```python
from build123d import *

# Parameters (mm, degrees)
SKETCH_1_R          = 14
EXTRUDE_1_DEPTH     = 19
SKETCH_2_W          = 13.202760332
SKETCH_2_H          = 6.2
EXTRUDE_2_DEPTH     = 15
SKETCH_3_R          = 1.75
EXTRUDE_3_DEPTH     = 1
SKETCH_4_R          = 4
EXTRUDE_4_DEPTH     = 1.8
SKETCH_5_R          = 2.5
EXTRUDE_5_DEPTH     = 8.2
CUT_EXTRUDE_START   = -6
CUT_EXTRUDE_1_DEPTH = 6


with BuildPart() as part:
    # 草图1 → 凸台-拉伸1 (new body)
    with BuildSketch(Plane(origin=(0, 0, 0), x_dir=(1, 0, 0), z_dir=(0, 1, 0))):
        with Locations(Location((0, 0, 0), (0, 0, 270))):
            Circle(SKETCH_1_R)
    extrude(amount=EXTRUDE_1_DEPTH)

    # 草图2 → 凸台-拉伸2 (add)
    with BuildSketch(Plane(origin=(0, 19, 0), x_dir=(1, 0, 0), z_dir=(0, 1, 0))):
        with Locations((0, -14)):
            Rectangle(SKETCH_2_W, SKETCH_2_H)
    extrude(amount=-EXTRUDE_2_DEPTH)

    # 草图3 → 凸台-拉伸3 (add)
    with BuildSketch(Plane(origin=(0, 19, 0), x_dir=(1, 0, 0), z_dir=(0, 1, 0))):
        with BuildLine():
            Line((17.5, -4), (-17.5, -4))
            ThreePointArc((-17.5, -4), (-21.5, 0), (-17.5, 4))
            Line((-17.5, 4), (17.5, 4))
            ThreePointArc((17.5, 4), (21.5, 0), (17.5, -4))
        make_face()
        with Locations(Location((-17.5, 0, 0), (0, 0, 270))):
            Circle(SKETCH_3_R, mode=Mode.SUBTRACT)
        with Locations(Location((17.5, 0, 0), (0, 0, 270))):
            Circle(SKETCH_3_R, mode=Mode.SUBTRACT)
    extrude(amount=-EXTRUDE_3_DEPTH)

    # 草图4 → 凸台-拉伸4 (add)
    with BuildSketch(Plane(origin=(0, 19, 0), x_dir=(1, 0, 0), z_dir=(0, 1, 0))):
        with Locations(Location((0, 6, 0), (0, 0, 270))):
            Circle(SKETCH_4_R)
    extrude(amount=EXTRUDE_4_DEPTH)

    # 草图5 → 凸台-拉伸5 (add)
    with BuildSketch(Plane(origin=(0, 20.8, 0), x_dir=(1, 0, 0), z_dir=(0, 1, 0))):
        with Locations(Location((0, 6, 0), (0, 0, 270))):
            Circle(SKETCH_5_R)
    extrude(amount=EXTRUDE_5_DEPTH)

    # 草图6 → 切除-拉伸1 (cut)
    with BuildSketch(Plane(origin=(0, 29, 0), x_dir=(1, 0, 0), z_dir=(0, 1, 0)).offset(CUT_EXTRUDE_START)):
        with BuildLine():
            Line((2, 4.5), (-2, 4.5))
            ThreePointArc((-2, 4.5), (0, 3.5), (2, 4.5))
        make_face()
        with BuildLine():
            Line((-2, 7.5), (2, 7.5))
            ThreePointArc((2, 7.5), (0, 8.5), (-2, 7.5))
        make_face()
    extrude(amount=CUT_EXTRUDE_1_DEPTH, mode=Mode.SUBTRACT)


solid = part.part
```
The model under review builds one solid part; all positions refer to its coordinate system, in mm. A direction names the side the tool comes from. Round coordinates to 2 decimals unless told otherwise and drop trailing zeros. Write each loop counter-clockwise with the first axis right and the second up, starting at its lowest first coordinate (ties: lowest second). Pieces come first, ordered by that corner, then holes.
(1) Machinability: for faces 4 (the cylindrical face through (-3.905, 19.887, -6.867)), 5 (the flat face through (0, 26, -7.5)), 6 (the flat face through (-15.5, 18.5, -4)), which of the approach directions +Z, -Z, +X, -X, +Y, -Y give a long, thin tool a straight path to every point of the face, cutting with its end or side? Answer none if there is none.
(2) We need section C-C on z = -6. Give the boundary of the cut face in (x, y).
(3) Mouldability with a two-part tool opening along Z and no side actions: class faces 1 (the cylindrical face through (2.11, 23.93, -4.66)), 2 (the cylindrical face through (19.235, 18.507, -0.228)), 3 (the flat face through (-15.4, 18.5, 4)) as +Z half, -Z half, draft (parallel to the pull), parting line (faces both ways), or undercut.
(4) We need section A-A on z = 0. Give the boundary of the cut face in (x, y).
(5) We need section B-B on x = 0. Give the boundary of the cut face in (y, z).
(6) We need section D-D on z = 6.5. Give the boundary of the cut face in (x, y), and give its area (3 significant figures).
(7) Wall thickness on L1, parallel to X at y = 18.5, z = 0; L2, parallel to Y at x = -12, z = 3; L3, parallel to X at y = 4.5, z = -10: over which ranges is each line inside the solid? List them lowest first.
(8) Insertion check: pin 1 (2 mm diameter, centred on y = 11.5, z = 2, fed in from -X); pin 2 (0.5 mm diameter, centred on x = 0, z = -8, fed in from +Y); pin 3 (0.8 mm diameter, centred on x = 14.5, y = 18.5, fed in from +Z). Each pin has a flat end and moves straight along its axis. Give the tip position at first contact, or say it passes through.
Findings below:
1. face 4: +Y
1. face 5: -Z, +X, -X, +Y
1. face 6: -Z, -X, +Y, -Y
2. outline: (-12.65, 0) - (12.65, 0) - (12.65, 19) - (4, 19) - (4, 20.8) - (2.5, 20.8) - (2.5, 29) - (-2.5, 29) - (-2.5, 20.8) - (-4, 20.8) - (-4, 19) - (-12.65, 19) - close
3. face 1: parting line
3. face 2: undercut
3. face 3: +Z half
4. outline: (-21.5, 18) - (-19.25, 18) - (-19.25, 19) - (-21.5, 19) - close; (-15.75, 18) - (-14, 18) - (-14, 0) - (14, 0) - (14, 18) - (15.75, 18) - (15.75, 19) - (-15.75, 19) - close; (19.25, 18) - (21.5, 18) - (21.5, 19) - (19.25, 19) - close
5. outline: (0, -14) - (19, -14) - (19, -10) - (20.8, -10) - (20.8, -8.5) - (23, -8.5) - (23, -7.5) - (29, -7.5) - (29, -4.5) - (23, -4.5) - (23, -3.5) - (20.8, -3.5) - (20.8, -2) - (19, -2) - (19, 17.1) - (4, 17.1) - (4, 14) - (0, 14) - close
6. outline: (-12.4, 0) - (12.4, 0) - (12.4, 19) - (-12.4, 19) - close
6. area: 471 mm2
7. L1: x = -21.5 to -19.25, -15.75 to 15.75, 19.25 to 21.5
7. L2: y = 0 to 19
7. L3: x = -9.8 to 9.8
8. pin 1: stops at x = -13.96
8. pin 2: stops at y = 23
8. pin 3: stops at z = 4
